from build123d import *

# Parameters (mm, degrees)
SKETCH_2_R      = 28.5
SKETCH_2_R_2    = 15
SKETCH_2_R_3    = 1.6
EXTRUDE_1_DEPTH = 3
EXTRUDE_START   = -3
SKETCH_4_R      = 1.6
EXTRUDE_2_DEPTH = 3


with BuildPart() as part:
    # 草图2 → 凸台-拉伸1 (new body)
    with BuildSketch(Plane.XY):
        Circle(SKETCH_2_R)
        Circle(SKETCH_2_R_2, mode=Mode.SUBTRACT)
        with Locations((0, 19)):
            Circle(SKETCH_2_R_3, mode=Mode.SUBTRACT)
        with Locations((13.435028843, 13.435028843)):
            Circle(SKETCH_2_R_3, mode=Mode.SUBTRACT)
        with Locations((19, 0)):
            Circle(SKETCH_2_R_3, mode=Mode.SUBTRACT)
        with Locations((13.435028843, -13.435028843)):
            Circle(SKETCH_2_R_3, mode=Mode.SUBTRACT)
        with Locations((0, -19)):
            Circle(SKETCH_2_R_3, mode=Mode.SUBTRACT)
        with Locations((-13.435028843, -13.435028843)):
            Circle(SKETCH_2_R_3, mode=Mode.SUBTRACT)
        with Locations((-19, 0)):
            Circle(SKETCH_2_R_3, mode=Mode.SUBTRACT)
        with Locations((-13.435028843, 13.435028843)):
            Circle(SKETCH_2_R_3, mode=Mode.SUBTRACT)
    extrude(amount=EXTRUDE_1_DEPTH)

    # 草图4 → 凸台-拉伸2 (add)
    with BuildSketch(Plane.XY.offset(3).offset(EXTRUDE_START)):
        with BuildLine():
            Line((-36.339888851, -5.595677643), (-19.093416125, -21.158720677))
            ThreePointArc((-19.093416125, -21.158720677), (-17.803808855, 22.254761069), (24.833892005, 13.983125827))
            Line((24.833892005, 13.983125827), (13.573611336, 33.981271988))
            ThreePointArc((13.573611336, 33.981271988), (12.840202642, 34.726636032), (11.830882073, 35))
            Line((11.830882073, 35), (-35, 35))
            ThreePointArc((-35, 35), (-36.414213562, 34.414213562), (-37, 33))
            Line((-37, 33), (-37, -4.110855139))
            ThreePointArc((-37, -4.110855139), (-36.827536279, -4.923327384), (-36.339888851, -5.595677643))
        make_face()
        with Locations((-31, 30)):
            Circle(SKETCH_4_R, mode=Mode.SUBTRACT)
        with Locations((-31, 10)):
            Circle(SKETCH_4_R, mode=Mode.SUBTRACT)
        with Locations((-22, 32)):
            Circle(SKETCH_4_R, mode=Mode.SUBTRACT)
        with Locations((-2, 32)):
            Circle(SKETCH_4_R, mode=Mode.SUBTRACT)
    extrude(amount=EXTRUDE_2_DEPTH)


solid = part.part
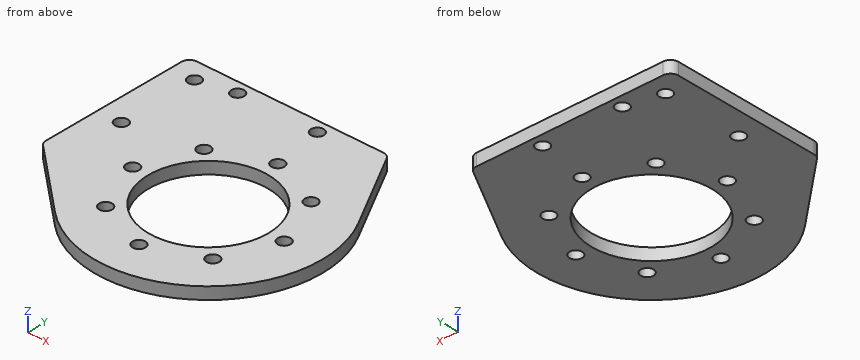
For this review, take the finished solid that the model builds, in its own axes (mm). Coordinates: 2 decimals unless noted, no trailing zeros. Order: outer loops, then holes, each group sorted by start corner. A loop starts at its lowest first (then second) coordinate and runs counter-clockwise, first axis right, second up. Notation, with made-up numbers: (-14.75, -35) - (4.25, -35) arc R14 cw to (4.25, -27) - close; hole circle Ø10 at (43, 16.25). An arc over 180 degrees is marked (long way). Use one line per item in the form item = value.
Q1. Consider section D-D (x = -31). Give the boundary of the cut face in (y, z), then the cut area to 3 significant figures.
Checked values:
outline = (-10.41, 0) - (8.4, 0) - (8.4, 3) - (-10.41, 3) - close; (11.6, 0) - (28.4, 0) - (28.4, 3) - (11.6, 3) - close; (31.6, 0) - (35, 0) - (35, 3) - (31.6, 3) - close
area = 117 mm2
Q2. Consider section B-B (y = -10.5). Give the boundary of the cut face in (x, z), then the cut area to 3 significant figures.
Checked values:
outline = (-30.91, 0) - (-10.71, 0) - (-10.71, 3) - (-30.91, 3) - close; (10.71, 0) - (26.5, 0) - (26.5, 3) - (10.71, 3) - close
area = 108 mm2
Q3. For P1, Ø1, axis at x = 19.5, z = 0.5, coming from the -Y side; P2, Ø3, axis at x = -31, y = 10, coming from the -Z side; P3, Ø3.5, axis at x = -2, y = 32, coming from the +Z side, all flat-tipped, find the tip position at first contact; note any pin that passes through.
Checked values:
P1 = -21.24
P2 = through
P3 = 3
Q4. For probe 1 along Y at (x, z) = (-2, 1.9); probe 2 along Y at (x, z) = (-31, 1.8); probe 3 along X at (y, z) = (-1, 0.85), list the stretches that pass through material, from the lowest coordinate up. Write a range as from..to.
Checked values:
probe_1 = -28.43..-14.87, 14.87..30.4, 33.6..35
probe_2 = -10.41..8.4, 11.6..28.4, 31.6..35
probe_3 = -37..-20.25, -17.75..-14.97, 14.97..17.75, 20.25..28.48
Q5. Consider section C-C (y = 10). Give the boundary of the cut face in (x, z), then the cut area to 3 significant figures.
Checked values:
outline = (-37, 0) - (-32.6, 0) - (-32.6, 3) - (-37, 3) - close; (-29.4, 0) - (-11.18, 0) - (-11.18, 3) - (-29.4, 3) - close; (11.18, 0) - (26.69, 0) - (26.69, 3) - (11.18, 3) - close
area = 114 mm2
Q6. Consider section A-A (x = -22). Give the boundary of the cut face in (y, z), then the cut area to 3 significant figures.
Checked values:
outline = (-18.54, 0) - (30.4, 0) - (30.4, 3) - (-18.54, 3) - close; (33.6, 0) - (35, 0) - (35, 3) - (33.6, 3) - close
area = 151 mm2
